Design review of the part built by this model. Coordinates are the model's own, in mm. Round coordinates to 2 decimals unless told otherwise and drop trailing zeros. Order: outer loops, then holes, each group sorted by start corner. A loop starts at its lowest first (then second) coordinate and runs counter-clockwise, first axis right, second up. Notation, with made-up numbers: M 51.5,10 L 91.5,10 A18 cw 91.5,37 Z; hole C 9.25,49.25 d9. An arc over 180 degrees is marked long. Write each question's results on one line, items separated by ' | '. Start each with the question number.
Item 1: The part is to be moulded in two halves that separate along X. For faces 1 (the flat face through (21, 2, -5)), 2 (the cylindrical face through (47.52, 1.57, 48.55)), 3 (the cylindrical face through (-2.66, 1.57, 44.92)), say which applies: +X half, -X half, draft (parallel to the pull), parting line (faces both ways), or undercut.
Item 2: Take a section at C-C, the plane x = 20.07. Write out the cut boundary in (y, z) (3 decimals).
Item 3: Take a section at D-D, the plane y = 2.3. Count the separate pieces of the cut face and the enclosed holes in it, plus the area to 3 significant figures.
Item 4: Wall thickness on line 1 (X direction, y = 1.05, z = 7); line 2 (X direction, y = 0.4, z = 26.5); line 3 (Z direction, x = 4.5, y = 0.65): over which ranges is each line inside the solid? List them lowest first. Write a range as [from, to].
Item 5: Clearance check with a flat-ended pin moving along its axis: pin 1 (6 mm diameter, centred on x = 23, z = 34.5, fed in from -Y). State where the tip first meets the part, or that it passes through.
Item 6: Take a section at B-B, the plane x = 35. Write out the cut boundary in (y, z) (3 decimals), plus the area to 3 significant figures.
Item 7: Take a section at A-A, the plane z = 28. Write out the cut boundary in (x, y) (3 decimals).
```python
from build123d import *

# Parameters (mm, degrees)
SKETCH1_W             = 42
SKETCH1_H             = 54
SKETCH1_R             = 1.6
SKETCH1_R_2           = 1.75
BOSS_EXTRUDE1_DEPTH   = 3.175
SKETCH2_W             = 6
SKETCH2_H             = 54
BOSS_EXTRUDE2_DEPTH   = 3.175
F_4_40_TAPPED_HOLE1_D = 2.2606
FILLET1_R             = 1.5875


with BuildPart() as part:
    # Sketch1 → Boss-Extrude1 (new body)
    with BuildSketch(Plane(origin=(0, 0, 0), x_dir=(1, 0, 0), z_dir=(0, 1, 0))):
        with Locations((21, -22)):
            Rectangle(SKETCH1_W, SKETCH1_H)
        with Locations(Location((35, -7, 0), (0, 0, 270))):
            Circle(SKETCH1_R, mode=Mode.SUBTRACT)
        with Locations(Location((5, -37, 0), (0, 0, 270))):
            Circle(SKETCH1_R, mode=Mode.SUBTRACT)
        with Locations(Location((20.07, -28, 0), (0, 0, 270))):
            Circle(SKETCH1_R_2, mode=Mode.SUBTRACT)
        with Locations(Location((35, -37, 0), (0, 0, 270))):
            Circle(SKETCH1_R, mode=Mode.SUBTRACT)
        with Locations(Location((40.07, -28, 0), (0, 0, 270))):
            Circle(SKETCH1_R_2, mode=Mode.SUBTRACT)
        with Locations(Location((5, -7, 0), (0, 0, 270))):
            Circle(SKETCH1_R, mode=Mode.SUBTRACT)
    extrude(amount=BOSS_EXTRUDE1_DEPTH)

    # Sketch2 → Boss-Extrude2 (add)
    with BuildSketch(Plane(origin=(0, 3.175, 0), x_dir=(1, 0, 0), z_dir=(0, 1, 0))):
        with Locations((-3, -22)):
            Rectangle(SKETCH2_W, SKETCH2_H)
        with Locations((45, -22)):
            Rectangle(SKETCH2_W, SKETCH2_H)
    extrude(amount=-BOSS_EXTRUDE2_DEPTH)

    # #4-40 Tapped Hole1 (through all)
    with Locations(Plane(origin=(-3, 3.175, -2), x_dir=(0, 0, 1), z_dir=(0, 1, 0))):
        with Locations((0, 0), (48, 0), (0, 48), (48, 48)):
            Hole(F_4_40_TAPPED_HOLE1_D / 2)

    # Fillet1
    fillet1_edges = [part.edges().sort_by_distance(p)[0] for p in [
        (-6, 1.5875, -5),
        (-6, 1.5875, 49),
        (48, 1.5875, 49),
        (48, 1.5875, -5),
    ]]
    fillet(fillet1_edges, radius=FILLET1_R)


solid = part.part
```
Results list:
1) face 1: draft | face 2: +X half | face 3: undercut
2) outline: M 0,-5 L 3.175,-5 L 3.175,26.25 L 0,26.25 Z; M 0,29.75 L 3.175,29.75 L 3.175,49 L 0,49 Z
3) separate pieces: 1 | enclosed holes: 10 | area: 2,850 mm²
4) line 1: [-6, 3.4], [6.6, 33.4], [36.6, 48] | line 2: [-6, 19.17], [20.97, 39.17], [40.97, 48] | line 3: [-5, 5.48], [8.52, 35.48], [38.52, 49]
5) pin 1: y = 0
6) outline: M 0,-5 L 3.175,-5 L 3.175,5.4 L 0,5.4 Z; M 0,8.6 L 3.175,8.6 L 3.175,35.4 L 0,35.4 Z; M 0,38.6 L 3.175,38.6 L 3.175,49 L 0,49 Z | area: 151 mm²
7) outline: M -6,0 L 18.32,0 L 18.32,3.175 L -6,3.175 Z; M 21.82,0 L 38.32,0 L 38.32,3.175 L 21.82,3.175 Z; M 41.82,0 L 48,0 L 48,3.175 L 41.82,3.175 Z
